Autodesk Inventor part; units mm, degrees
ref_plane "YZ Plane" through (0, 0, 0) normal (1, 0, 0) x (0, 1, 0)
ref_plane "XZ Plane" through (0, 0, 0) normal (0, 1, 0) x (-1, 0, 0)
ref_plane "XY Plane" through (0, 0, 0) normal (0, 0, 1) x (1, 0, 0)
sketch "Sketch1" plane through (0, 0, 0) normal (0, 0, 1) x (1, 0, 0)
  line L0 (0, 0) -> (-19, 0)
  line L1 (-19, 0) -> (-19, 0)
  line L2 (-19, 0) -> (-109, 0)
  line L3 (-109, 0) -> (-109, 3)
  line L4 (-109, 3) -> (-17, 3)
  line L5 (-17, 3) -> (-17, 3)
  line L6 (-17, 3) -> (0, 3)
  line L7 (0, 3) -> (0, 0)
  dimension "d1" = 0
  dimension "d3" = 3
  dimension "d4" = 3
  dimension "d5" = 17
  dimension "d6" = 2
  dimension "d7" = 90
extrude "Extrusion1" add sketch "Sketch1" along normal blind 6
chamfer "Chamfer1" distance 2 angle 45 2 edges at (0, 1.5, 0) (0, 1.5, 6)
sketch "Sketch3" plane through (-109, 0, 0) normal (-1, 0, 0) x (0, 0, 1)
  line L0 (3, 0) -> (3, 4.5868) construction
  line L1 (0.8, 1.5) -> (1.5, 0)
  line L2 (1.5, 0) -> (4.5, 0)
  line L3 (4.5, 0) -> (5.2, 1.5)
  line L4 (5.2, 1.5) -> (0.8, 1.5)
  line L5 (0, 0) -> (6, 0)
  point P0 (0, 0)
  dimension "d20" = 1.5
  dimension "d21" = 2.2
  dimension "d22" = 4.4
  dimension "d23" = 3
  dimension "d24" = 1.5
extrude "Extrusion3" cut sketch "Sketch3" against normal blind 87
sketch "Sketch4" plane through (-109, 3, 6) normal (0, 1, 0) x (1, 0, 0)
  line L0 (109, 4) -> (109, 2)
  line L1 (109, 3) -> (86.5142, 3) construction
  circle A0 centre (96.5, 3) radius 0.75
  circle A1 centre (105.5, 3) radius 0.75
  point P0 (109, 6)
  dimension "d42" = 3.5
  dimension "d43" = 9
  dimension "d44" = 1.5
  dimension "d45" = 1.5
extrude "Extrusion4" cut sketch "Sketch4" against normal through all
equation "\"d20\" = 0.5 * d23"
equation "\"d21\" = 0.5 * d22"
properties part number "spazzola - asta"
Design review of the part built by this model. Coordinates are the model's own, in mm. Coordinates: 2 decimals unless noted, no trailing zeros. Order: outer loops, then holes, each group sorted by start corner. A loop starts at its lowest first (then second) coordinate and runs counter-clockwise, first axis right, second up. Notation, with made-up numbers: M 66.5,5 L 83.5,5 A26 ccw 83.5,31 Z; hole C 50.5,-34 d9. An arc over 180 degrees is marked long. Use a Markdown table: item, result.
(1) For P1, Ø1.5, axis at x = -79.5, y = 2, coming from the -Z side; P2, Ø0.5, axis at y = 0.5, z = 3.5, coming from the -X side, all flat-tipped, find the tip position at first contact; note any pin that passes through.
Worked answers:
| item | result |
|---|---|
| P1 | stops at z = 0 |
| P2 | stops at x = -22 |
(2) Wall thickness on probe 1 along X at (y, z) = (0.7, 3); probe 2 along X at (y, z) = (1.75, 3); probe 3 along Z at (x, y) = (-3.5, 0.85): over which ranges is each line inside the solid? List them lowest first.
Worked answers:
| item | result |
|---|---|
| probe 1 | x = -22 to -13.25, -11.75 to -4.25, -2.75 to 0 |
| probe 2 | x = -109 to -13.25, -11.75 to -4.25, -2.75 to 0 |
| probe 3 | z = 0 to 2.25, 3.75 to 6 |
(3) Draft analysis for pull direction Z (two halves, no side actions). For faces 1 (the flat face through (-56, 2, 0)), 2 (the flat face through (-109, 2, 3)), 3 (the flat face through (-66, 1.5, 3)), state which applies: released by +Z, released by -Z, zero draft, split by the parting line, or undercut.
Worked answers:
| item | result |
|---|---|
| face 1 | released by -Z |
| face 2 | zero draft |
| face 3 | undercut |
(4) Add section A-A (x = -45.5). Give the boundary of the cut face in (y, z), then the cut area to 4 significant figures.
Worked answers:
| item | result |
|---|---|
| outline | M 0,0 L 3,0 L 3,6 L 0,6 L 0,4.5 L 1.5,5.2 L 1.5,0.8 L 0,1.5 Z |
| area | 12.45 mm2 |
(5) Add section B-B (y = 0.7). Give the boundary of the cut face in (x, z).
Worked answers:
| item | result |
|---|---|
| outline | M -109,0 L -2,0 L 0,2 L 0,4 L -2,6 L -109,6 L -109,4.83 L -22,4.83 L -22,1.17 L -109,1.17 Z; hole C -12.5,3 d1.5; hole C -3.5,3 d1.5 |
